Model file for the job. Use its own axes, mm. A direction names the side the tool comes from. Round coordinates to 2 decimals unless told otherwise and drop trailing zeros. Order: outer loops, then holes, each group sorted by start corner. A loop starts at its lowest first (then second) coordinate and runs counter-clockwise, first axis right, second up. Notation, with made-up numbers: (9.25, 56.5) - (68.25, 56.5) arc R19 cw to (68.25, 60.5) - close; hole circle Ø3 at (27, -30.75). An arc over 180 degrees is marked (long way). Put each result on its own line as item: value. Start each with the question number.
Item 1: Saw through at D-D on z = 1.6. List the corners of the cut face in (x, y).
Item 2: Saw through at B-B on z = 4.75. List the corners of the cut face in (x, y), plus the area to 3 significant figures.
Item 3: Saw through at C-C on y = 9.5. List the corners of the cut face in (x, z), plus the area to 3 significant figures.
Item 4: Probe probe 1 along X at (y, z) = (18, 5.2); probe 2 along X at (y, z) = (27.25, 3.15); probe 3 along Y at (x, z) = (24, 0.8). List the from-to ranges inside material, lowest first.
Item 5: Mould opens along Y. For faces 1 (the face through (0, 15, 3)), 2 (the face through (29.43, 29.4, 2.84)), 3 (the face through (3.5, 15, 4)) say: pulls with the +Y half, pulls with the -Y half, needs draft (parallel to the pull), parting line crosses it, or undercut.
Item 6: Pin check, flat tip, straight feed: pin 1 Ø2 at (x, y) = (5.5, 20) entering from +Z. Stop position of the tip, or through.
Item 7: Which spindle directions (+Z, -Z, +X, -X, +Y, -Y) get a long thin tool onto all of the face, cutting with end or side? Do faces 4 (the face through (0.6, 29.43, 2.84)), 5 (the face through (5, 15, 1)), 6 (the face through (6.923, 28.485, 3.775)). Say none if no direction does.
Item 8: Saw through at A-A on x = 7. List the corners of the cut face in (y, z).
Autodesk Fusion 360 part; units mm, degrees
sketch "Sketch1" plane through (0, 0, 0) normal (0, 0, 1) x (1, 0, 0)
  line L0 (0, 0) -> (30, 0)
  line L1 (30, 0) -> (30, 30)
  line L2 (30, 30) -> (0, 30)
  line L3 (0, 30) -> (0, 0)
  line L4 (7, 30) -> (7, 0) construction
  line L5 (23, 30) -> (23, 0) construction
  line L6 (15, 30) -> (15, 0) construction
  line L7 (3.5, 24.986) -> (3.5, 4.986)
  line L8 (10.5, 24.986) -> (10.5, 4.986)
  arc A0 (10.5, 24.986) -> (3.5, 24.986) centre (7, 24.986) ccw
  arc A1 (3.5, 4.986) -> (10.5, 4.986) centre (7, 4.986) ccw
  line L9 (5, 24.9854) -> (5, 4.9865)
  line L10 (9, 24.986) -> (9, 4.986)
  arc A2 (9, 24.986) -> (5, 24.9854) centre (7, 24.986) ccw
  arc A3 (5, 4.9865) -> (9, 4.986) centre (7, 4.986) ccw
  line L11 (26.5, 24.986) -> (26.5, 4.986)
  line L12 (25, 24.9854) -> (25, 4.9865)
  arc A4 (25, 24.9854) -> (21, 24.986) centre (23, 24.986) ccw
  arc A5 (21, 4.986) -> (25, 4.9865) centre (23, 4.986) ccw
  arc A6 (26.5, 24.986) -> (19.5, 24.986) centre (23, 24.986) ccw
  line L13 (19.5, 24.986) -> (19.5, 4.986)
  line L14 (21, 24.986) -> (21, 4.986)
  arc A7 (19.5, 4.986) -> (26.5, 4.986) centre (23, 4.986) ccw
  point P0 (7, 21.986)
  point P1 (23, 21.9825)
  point P2 (23.0012, 7.9825)
  point P3 (7.0013, 7.986)
  point P4 (23, 21.986)
  point P5 (22.9987, 7.986)
  dimension "d1" = 30
  dimension "d2" = 30
  dimension "d3" = 16
  dimension "d4" = 14
  dimension "d5" = 7
  dimension "d6" = 3
  dimension "d7" = 14
  dimension "d8" = 16
  dimension "d9" = 7
  dimension "d10" = 3
  dimension "d11" = 7
  dimension "d12" = 4
  dimension "d13" = 4
  dimension "d14" = 4
extrude "Extrude1" add sketch "Sketch1" along normal blind 6 contours L0 L1 L2 L3
extrude "Extrude2" add sketch "Sketch1" along normal blind 2 contours L7 L8 A0 A1 | L11 A6 L13 A7
fillet "Fillet1" radius 2 4 edges at (0, 0, 3) (30, 0, 3) (30, 30, 3) (0, 30, 3)
fillet "Fillet1" radius 0.4 1 faces at (13.5, 11.6527, 6)
Results found:
1. outline: (0, 2) arc R2 ccw to (2, 0) - (28, 0) arc R2 ccw to (30, 2) - (30, 28) arc R2 ccw to (28, 30) - (2, 30) arc R2 ccw to (0, 28) - close; hole (5, 4.99) arc R2 ccw to (9, 4.99) - (9, 24.99) arc R2 ccw to (5, 24.99) - close; hole (21, 4.99) arc R2 ccw to (25, 4.99) - (25, 24.99) arc R2 ccw to (21, 24.99) - close
2. outline: (0, 2) arc R2 ccw to (2, 0) - (28, 0) arc R2 ccw to (30, 2) - (30, 28) arc R2 ccw to (28, 30) - (2, 30) arc R2 ccw to (0, 28) - close; hole (3.5, 4.99) arc R3.5 ccw to (10.5, 4.99) - (10.5, 24.99) arc R3.5 ccw to (3.5, 24.99) - close; hole (19.5, 4.99) arc R3.5 ccw to (26.5, 4.99) - (26.5, 24.99) arc R3.5 ccw to (19.5, 24.99) - close
2. area: 540 mm²
3. outline: (0, 0) - (5, 0) - (5, 2) - (3.5, 2) - (3.5, 5.6) arc R0.4 ccw to (3.1, 6) - (0.4, 6) arc R0.4 ccw to (0, 5.6) - close; (9, 0) - (21, 0) - (21, 2) - (19.5, 2) - (19.5, 5.6) arc R0.4 ccw to (19.1, 6) - (10.9, 6) arc R0.4 ccw to (10.5, 5.6) - (10.5, 2) - (9, 2) - close; (25, 0) - (30, 0) - (30, 5.6) arc R0.4 ccw to (29.6, 6) - (26.9, 6) arc R0.4 ccw to (26.5, 5.6) - (26.5, 2) - (25, 2) - close
3. area: 108 mm²
4. probe 1: x = 0 to 3.5, 10.5 to 19.5, 26.5 to 30
4. probe 2: x = 0 to 4.33, 9.67 to 20.33, 25.67 to 30
4. probe 3: y = 0 to 3.25, 26.72 to 30
5. face 1: needs draft
5. face 2: pulls with the +Y half
5. face 3: undercut
6. pin 1: stops at z = 2
7. face 4: +Z, -Z, -X, +Y
7. face 5: +Z, -Z
7. face 6: +Z
8. outline: (0, 0) - (2.99, 0) - (2.99, 2) - (1.49, 2) - (1.49, 5.6) arc R0.4 ccw to (1.09, 6) - (0.4, 6) arc R0.4 ccw to (0, 5.6) - close; (26.99, 0) - (30, 0) - (30, 5.6) arc R0.4 ccw to (29.6, 6) - (28.89, 6) arc R0.4 ccw to (28.49, 5.6) - (28.49, 2) - (26.99, 2) - close
